Can you work these out from the model? Positions are in its coordinate system, mm. A direction names the side the tool comes from. Give positions to 0.01 mm unless a question says otherwise; leave off trailing zeros. Loops run counter-clockwise (first coordinate to the right, second up) from the corner with the lowest first, then second, coordinate; pieces in that order, holes last. Notation, with made-up numbers: (-38, -7) -> (5, -7) arc R31 ccw to (5, 20) -> close; hole circle Ø11 at (86.25, 41). An arc over 180 degrees is marked (long way). Return JSON: item names as keys, results as strings. Group by question number.
Q1. Suppose I cut it at D-D, the plane x = 8.5. Please give me the cut outline in (y, z) (3 decimals).
Q2. Which directions (+Z, -Z, +X, -X, +Y, -Y) give clear straight access to the entire face, cutting with the end or side of a thin tool? Please do faces 4 (the flat face through (15, -2, 7)), 5 (the flat face through (-15, 5, 1)), 6 (the cylindrical face through (0.18, -4.43, 12.4)), 7 (the flat face through (0, -15, 2)), 8 (the cylindrical face through (-12, -2, 6)).
Q3. I need wall thicknesses on line 1 along Y through (x, z) = (-2, 10); line 2 along X through (y, z) = (-13, 10.5); line 3 along Y through (x, z) = (-3.5, 4). Which ranges of each line are inside material? Lowest first, please. Write a range as [from, to].
Q4. Suppose I cut it at B-B, the plane z = 22. Please give me the cut outline in (x, y), and give its area (3 significant figures).
Q5. Suppose I cut it at C-C, the plane y = 19.5. Please give me the cut outline in (x, z).
Q6. Thinking about a two-plate mould opening in Y: for faces 1 (the cylindrical face through (12, -2, 6)), 2 (the flat face through (0, -2, 7.6)), 3 (the flat face through (-20.52, 18.584, 1.479)), which applies, pulls with the +Y half, pulls with the -Y half, needs draft (parallel to the pull), parting line crosses it, or undercut?
Q7. Suppose I cut it at A-A, the plane z = 6. Count the separate pieces of the cut face and the enclosed holes in it, and give its area (3 significant figures).
Q8. Will these pins go through, and if not, where does the flat tip stop? pin 1 (16 mm diameter, centred on x = 4, y = -10.5, fed in from +Z); pin 2 (1.5 mm diameter, centred on x = 4.5, z = 20.5, fed in from -Y); pin 3 (6 mm diameter, centred on y = -19.5, z = 28, fed in from +X).
```python
from build123d import *

# Parameters (mm, degrees)
F0_W      = 30
F0_H      = 10
F0_R      = 3
F1_DEPTH  = 3
F2_R      = 3
F3_DEPTH  = 30
F4_W      = 30
F4_H      = 5
F5_DEPTH  = 10
F7_DEPTH  = 5
F8_R      = 2
F10_DEPTH = 20


with BuildPart() as f1:
    # F0 (on Top) → F1 (new body)
    with BuildSketch(Plane.XY):
        with BuildLine():
            ThreePointArc((-43.277054, -7.431739), (-34.442413, -5.20991), (-29.2557, -12.69893))
            ThreePointArc((-29.2557, -12.69893), (-33.671529, -19.851113), (-42.04413, -19.107591))
            Line((-42.04413, -19.107591), (-6.405723, -45.735934))
            ThreePointArc((-6.405723, -45.735934), (-5.201464, -32.17509), (6.382707, -39.327273))
            ThreePointArc((6.382707, -39.327273), (6.065934, -41.556178), (5.140702, -43.608569))
            Line((5.140702, -43.608569), (41.625059, 13.981723))
            ThreePointArc((41.625059, 13.981723), (26.999486, 16.813462), (39.655494, 24.671681))
            Line((39.655494, 24.671681), (12.418684, 45.022509))
            ThreePointArc((12.418684, 45.022509), (14.782437, 42.198018), (15.630254, 38.613848))
            ThreePointArc((15.630254, 38.613848), (4.816967, 31.124828), (1.6089, 43.881039))
            Line((1.6089, 43.881039), (-43.277054, -7.431739))
        make_face()
        with Locations((0, 5)):
            Rectangle(F0_W, F0_H, mode=Mode.SUBTRACT)
        with BuildLine():
            ThreePointArc((-42.04413, -19.107591), (-33.671529, -19.851113), (-29.2557, -12.69893))
            ThreePointArc((-29.2557, -12.69893), (-34.442413, -5.20991), (-43.277054, -7.431739))
            ThreePointArc((-43.277054, -7.431739), (-45.211467, -13.539027), (-42.04413, -19.107591))
        make_face()
        with Locations((-37.2557, -12.69893)):
            Circle(F0_R, mode=Mode.SUBTRACT)
        with BuildLine():
            ThreePointArc((12.418684, 45.022509), (6.790157, 46.569615), (1.6089, 43.881039))
            ThreePointArc((1.6089, 43.881039), (4.816967, 31.124828), (15.630254, 38.613848))
            ThreePointArc((15.630254, 38.613848), (14.782437, 42.198018), (12.418684, 45.022509))
        make_face()
        with Locations((7.630254, 38.613848)):
            Circle(F0_R, mode=Mode.SUBTRACT)
        with BuildLine():
            ThreePointArc((42.867064, 18.26302), (42.019246, 21.84719), (39.655494, 24.671681))
            ThreePointArc((39.655494, 24.671681), (26.999486, 16.813462), (41.625059, 13.981723))
            ThreePointArc((41.625059, 13.981723), (42.550291, 16.034114), (42.867064, 18.26302))
        make_face()
        with Locations((34.867064, 18.26302)):
            Circle(F0_R, mode=Mode.SUBTRACT)
        with BuildLine():
            ThreePointArc((6.382707, -39.327273), (-5.201464, -32.17509), (-6.405723, -45.735934))
            ThreePointArc((-6.405723, -45.735934), (-0.167735, -47.19485), (5.140702, -43.608569))
            ThreePointArc((5.140702, -43.608569), (6.065934, -41.556178), (6.382707, -39.327273))
        make_face()
        with Locations((-1.617293, -39.327273)):
            Circle(F0_R, mode=Mode.SUBTRACT)
    extrude(amount=F1_DEPTH)

    # F2 (on face) → F3 (join)
    with BuildSketch(Plane.XY.offset(3)):
        with BuildLine():
            ThreePointArc((1.6089, 43.881039), (4.816967, 31.124828), (15.630254, 38.613848))
            ThreePointArc((15.630254, 38.613848), (14.782437, 42.198018), (12.418684, 45.022509))
            ThreePointArc((12.418684, 45.022509), (6.790157, 46.569615), (1.6089, 43.881039))
        make_face()
        with Locations((7.630254, 38.613848)):
            Circle(F2_R, mode=Mode.SUBTRACT)
        with BuildLine():
            ThreePointArc((-29.2557, -12.69893), (-34.442413, -5.20991), (-43.277054, -7.431739))
            ThreePointArc((-43.277054, -7.431739), (-45.211467, -13.539027), (-42.04413, -19.107591))
            ThreePointArc((-42.04413, -19.107591), (-33.671529, -19.851113), (-29.2557, -12.69893))
        make_face()
        with Locations((-37.2557, -12.69893)):
            Circle(F2_R, mode=Mode.SUBTRACT)
        with BuildLine():
            ThreePointArc((42.867064, 18.26302), (42.019246, 21.84719), (39.655494, 24.671681))
            ThreePointArc((39.655494, 24.671681), (26.999486, 16.813462), (41.625059, 13.981723))
            ThreePointArc((41.625059, 13.981723), (42.550291, 16.034114), (42.867064, 18.26302))
        make_face()
        with Locations((34.867064, 18.26302)):
            Circle(F2_R, mode=Mode.SUBTRACT)
        with BuildLine():
            ThreePointArc((-6.405723, -45.735934), (-0.167735, -47.19485), (5.140702, -43.608569))
            ThreePointArc((5.140702, -43.608569), (6.065934, -41.556178), (6.382707, -39.327273))
            ThreePointArc((6.382707, -39.327273), (-5.201464, -32.17509), (-6.405723, -45.735934))
        make_face()
        with Locations((-1.617293, -39.327273)):
            Circle(F2_R, mode=Mode.SUBTRACT)
    extrude(amount=F3_DEPTH)

    # F4 (on face) → F5 (join)
    with BuildSketch(Plane.XY.offset(3)):
        with Locations((0, -2.5)):
            Rectangle(F4_W, F4_H)
    extrude(amount=F5_DEPTH)

    # F6 (on face) → F7 (cut, through all)
    with BuildSketch(Plane(origin=(0, 0, 0), x_dir=(-1, 0, 0), z_dir=(0, 1, 0))):
        with BuildLine():
            Line((10.4, 7.6), (-10.4, 7.6))
            ThreePointArc((-10.4, 7.6), (-12, 6), (-10.4, 4.4))
            Line((-10.4, 4.4), (10.4, 4.4))
            ThreePointArc((10.4, 4.4), (12, 6), (10.4, 7.6))
        make_face()
    extrude(amount=-F7_DEPTH, mode=Mode.SUBTRACT)

    # F8
    f8_edges = [f1.edges().sort_by_distance(p)[0] for p in [
        (15, -5, 8),
        (15, -2.5, 13),
        (0, -5, 13),
        (-15, -5, 8),
        (-15, -2.5, 13),
    ]]
    fillet(f8_edges, radius=F8_R)

    # F9 (on face) → F10 (cut)
    with BuildSketch(Plane.XZ.offset(5)):
        with BuildLine():
            Line((10.4, 10), (-10.4, 10))
            ThreePointArc((-10.4, 10), (-11.785831, 9.752262), (-13, 9.039737))
            Line((-13, 9.039737), (-13, 3))
            Line((-13, 3), (13, 3))
            Line((13, 3), (13, 9.039737))
            ThreePointArc((13, 9.039737), (11.785831, 9.752262), (10.4, 10))
        make_face()
        with BuildLine():
            ThreePointArc((-10.4, 4.4), (-12, 6), (-10.4, 7.6))
            Line((-10.4, 7.6), (10.4, 7.6))
            ThreePointArc((10.4, 7.6), (12, 6), (10.4, 4.4))
            Line((10.4, 4.4), (-10.4, 4.4))
        make_face(mode=Mode.SUBTRACT)
        with BuildLine():
            Line((-13, 3), (-13, 9.039737))
            ThreePointArc((-13, 9.039737), (-14.152262, 4.614169), (-10.4, 2))
            Line((-10.4, 2), (10.4, 2))
            ThreePointArc((10.4, 2), (14.152262, 4.614169), (13, 9.039737))
            Line((13, 9.039737), (13, 3))
            Line((13, 3), (-13, 3))
        make_face()
    extrude(amount=F10_DEPTH, mode=Mode.SUBTRACT)


solid = f1.part
```
Ans:
{
 "1": {"outline": "(-38.306, 0) -> (0, 0) -> (0, 4.4) -> (-5, 4.4) -> (-5, 2) -> (-25, 2) -> (-25, 3) -> (-38.306, 3) -> close; (-5, 7.6) -> (0, 7.6) -> (0, 13) -> (-3, 13) arc R2 ccw to (-5, 11) -> close; (10, 0) -> (35.743, 0) -> (35.743, 33) -> (30.661, 33) -> (30.661, 3) -> (10, 3) -> close; (41.485, 0) -> (46.566, 0) -> (46.566, 33) -> (41.485, 33) -> close"},
 "2": {"face 4": "+Z, +X, -Y", "face 5": "+Z, -Z", "face 6": "+Z, +X", "face 7": "+Z", "face 8": "+Y, -Y"},
 "3": {"line 1": "y = [-47.32, -42.3], [-36.35, -31.34], [-5, 0]", "line 2": "x = [-45.25, -40.24], [-34.27, -29.26]", "line 3": "y = [-47.1, -41.66], [-36.99, -31.55], [-5, 0]"},
 "4": {"outline": "(-43.28, -7.43) arc R8 ccw to (-42.04, -19.11) arc R8 ccw (long way) to start; (-6.41, -45.74) arc R8 ccw to (5.14, -43.61) arc R8 ccw to (6.38, -39.33) arc R8 ccw (long way) to start; (1.61, 43.88) arc R8 ccw (long way) to (15.63, 38.61) arc R8 ccw to (12.42, 45.02) arc R8 ccw to start; (39.66, 24.67) arc R8 ccw (long way) to (41.63, 13.98) arc R8 ccw to (42.87, 18.26) arc R8 ccw to start; hole circle Ø6 at (-37.26, -12.7); hole circle Ø6 at (-1.62, -39.33); hole circle Ø6 at (7.63, 38.61); hole circle Ø6 at (34.87, 18.26)", "area": "691 mm^2"},
 "5": {"outline": "(-19.72, 0) -> (32.13, 0) -> (32.13, 33) -> (26.96, 33) -> (26.96, 3) -> (-19.72, 3) -> close; (37.6, 0) -> (42.77, 0) -> (42.77, 33) -> (37.6, 33) -> close"},
 "6": {"face 1": "needs draft", "face 2": "undercut", "face 3": "pulls with the +Y half"},
 "7": {"separate pieces": "6", "enclosed holes": "4", "area": "719 mm^2"},
 "8": {"pin 1": "stops at z = 13", "pin 2": "stops at y = -45.26", "pin 3": "stops at x = -30.22"}
}
